Source: CAD feature listing. Evaluate the final solid. Frame: model axes, mm. A direction names the side the tool comes from. Give positions to 0.01 mm unless a question says otherwise; leave off trailing zeros. Loops run counter-clockwise (first coordinate to the right, second up) from the corner with the lowest first, then second, coordinate; pieces in that order, holes last. Notation, with made-up numbers: (56, 78) -> (103, 78) arc R37 ccw to (103, 115) -> close; hole circle Ø8 at (25.5, 41.25). An arc over 180 degrees is marked (long way). Return JSON: item names as keys, results as strings. Group by question number.
(1) Cut plane B-B on z = 6.25. Give the number of separate pieces and of enclosed holes in the cut face, then the cut area to 3 significant figures.
(2) Ray query, line 1 (Y direction, x = -23, z = 1.75); line 2 (Y direction, x = -2, z = 9); line 3 (Y direction, x = 1.5, z = 9). Return the intervals inside material, ascending. Write a range as from..to.
(3) Draft query along X for faces 1 (the face through (-29.97, 1.32, 4.93)), 2 (the face through (0, 23, 5)), 3 (the face through (-25, 0, 20)), 4 (the face through (-1.25, -4, 5)). Return one class per face: released by +X, released by -X, zero draft, split by the parting line, or undercut.
(4) Pin query (flat end, axial travel): pin 1 (0.8 mm diameter, centred on y = 0.5, z = 6, fed in from +X); pin 2 (3 mm diameter, centred on y = -5.5, z = 3.5, fed in from -X); pin 3 (7 mm diameter, centred on x = 4.5, z = 6.5, fed in from -Y); pin 4 (3 mm diameter, centred on x = -16.5, z = 6.5, fed in from -Y). Return the tip coordinate at first contact, or that it passes through.
(5) Cut plane C-C on x = 9.5. Return loops of the section in (y, z), then the cut area to 3 significant figures.
(6) Cut plane D-D on x = -19. Return loops of the section in (y, z).
(7) Access query for faces 5 (the face through (1.25, -4, 5)), 6 (the face through (6, 7, 0)), 7 (the face through (-27.5, 0.1, 14.9)). Directions: +Z, -Z, +X, -X, +Y, -Y. A direction counts if a zero-diameter tool reaches every point of the face in a straight line with its end or side. Return the directions, or none.
(8) Cut plane A-A on x = 0. Return loops of the section in (y, z).
```python
from build123d import *

# Parameters (mm, degrees)
SKETCH_1_R          = 30
EXTRUDE_1_DEPTH     = 10
SKETCH_2_R          = 2.5
EXTRUDE_3_DEPTH     = 10
SKETCH_5_W          = 2.5
SKETCH_5_H          = 6.25
SKETCH_5_W_2        = 6.25
SKETCH_5_H_2        = 2.5
CUT_EXTRUDE_3_DEPTH = 10
CUT_EXTRUDE_4_DEPTH = 20


with BuildPart() as part:
    # 草图1 → 凸台-拉伸1 (new body)
    with BuildSketch(Plane.XY):
        Circle(SKETCH_1_R)
    extrude(amount=EXTRUDE_1_DEPTH)

    # 草图2 → 凸台-拉伸3 (add)
    with BuildSketch(Plane.XY.offset(10)):
        with Locations((-25, 0)):
            Circle(SKETCH_2_R)
    extrude(amount=EXTRUDE_3_DEPTH)

    # 草图5 → 切除-拉伸3 (cut)
    with BuildSketch(Plane.XY.offset(10)):
        with Locations((0, 4.375)):
            Rectangle(SKETCH_5_W, SKETCH_5_H)
        with Locations((-4.375, 0)):
            Rectangle(SKETCH_5_W_2, SKETCH_5_H_2)
        with Locations((4.375, 0)):
            Rectangle(SKETCH_5_W_2, SKETCH_5_H_2)
        with Locations((0, -4.375)):
            Rectangle(SKETCH_5_W, SKETCH_5_H)
        Rectangle(SKETCH_5_W, SKETCH_5_H_2)
    extrude(amount=-CUT_EXTRUDE_3_DEPTH, mode=Mode.SUBTRACT)

    # 草图7 → 切除-拉伸4 (cut)
    with BuildSketch(Plane.XY.offset(10)):
        with BuildLine():
            ThreePointArc((23.382685902, 13.5), (0, 27), (-23.382685902, 13.5))
            ThreePointArc((-23.382685902, 13.5), (-22.650635095, 10.767949192), (-19.918584287, 11.5))
            ThreePointArc((-19.918584287, 11.5), (0, 23), (19.918584287, 11.5))
            ThreePointArc((19.918584287, 11.5), (22.650635095, 10.767949192), (23.382685902, 13.5))
        make_face()
        with BuildLine():
            ThreePointArc((23.382685902, -13.5), (0, -27), (-23.382685902, -13.5))
            ThreePointArc((-23.382685902, -13.5), (-22.650635095, -10.767949192), (-19.918584287, -11.5))
            ThreePointArc((-19.918584287, -11.5), (0, -23), (19.918584287, -11.5))
            ThreePointArc((19.918584287, -11.5), (22.650635095, -10.767949192), (23.382685902, -13.5))
        make_face()
        with BuildLine():
            ThreePointArc((-8.5, 14.722431864), (-17, 0), (-8.5, -14.722431864))
            ThreePointArc((-8.5, -14.722431864), (-5.767949192, -13.990381057), (-6.5, -11.258330249))
            ThreePointArc((-6.5, -11.258330249), (-13, 0), (-6.5, 11.258330249))
            ThreePointArc((-6.5, 11.258330249), (-5.767949192, 13.990381057), (-8.5, 14.722431864))
        make_face()
        with BuildLine():
            ThreePointArc((8.5, 14.722431864), (17, 0), (8.5, -14.722431864))
            ThreePointArc((8.5, -14.722431864), (5.767949192, -13.990381057), (6.5, -11.258330249))
            ThreePointArc((6.5, -11.258330249), (13, 0), (6.5, 11.258330249))
            ThreePointArc((6.5, 11.258330249), (5.767949192, 13.990381057), (8.5, 14.722431864))
        make_face()
    extrude(amount=-CUT_EXTRUDE_4_DEPTH, mode=Mode.SUBTRACT)


solid = part.part
```
Answers:
{
 "1": {"separate pieces": "1", "enclosed holes": "5", "area": "2,040 mm²"},
 "2": {"line 1": "-19.26..-14.14, -11.02..11.02, 14.14..19.26", "line 2": "-29.93..-26.93, -22.91..-1.25, 1.25..22.91, 26.93..29.93", "line 3": "-29.96..-26.96, -22.95..-1.25, 1.25..22.95, 26.96..29.96"},
 "3": {"face 1": "split by the parting line", "face 2": "undercut", "face 3": "zero draft", "face 4": "undercut"},
 "4": {"pin 1": "x = 30", "pin 2": "x = -29.73", "pin 3": "y = -29.98", "pin 4": "y = -25.98"},
 "5": {"outline": "(-28.46, 0) -> (-25.27, 0) -> (-25.27, 10) -> (-28.46, 10) -> close; (-20.95, 0) -> (-14.1, 0) -> (-14.1, 10) -> (-20.95, 10) -> close; (-8.87, 0) -> (8.87, 0) -> (8.87, 10) -> (-8.87, 10) -> close; (14.1, 0) -> (20.95, 0) -> (20.95, 10) -> (14.1, 10) -> close; (25.27, 0) -> (28.46, 0) -> (28.46, 10) -> (25.27, 10) -> close", "area": "378 mm²"},
 "6": {"outline": "(-23.22, 0) -> (-19.18, 0) -> (-19.18, 10) -> (-23.22, 10) -> close; (-12.96, 0) -> (12.96, 0) -> (12.96, 10) -> (-12.96, 10) -> close; (19.18, 0) -> (23.22, 0) -> (23.22, 10) -> (19.18, 10) -> close"},
 "7": {"face 5": "+Z, -Z", "face 6": "-Z, +X, -X, +Y, -Y", "face 7": "+Z"},
 "8": {"outline": "(-30, 0) -> (-27, 0) -> (-27, 10) -> (-30, 10) -> close; (-23, 0) -> (-7.5, 0) -> (-7.5, 10) -> (-23, 10) -> close; (7.5, 0) -> (23, 0) -> (23, 10) -> (7.5, 10) -> close; (27, 0) -> (30, 0) -> (30, 10) -> (27, 10) -> close"}
}
